```python
from build123d import *

# Parameters (mm, degrees)
BOSS_EXTRUDE1_DEPTH      = 4.7625
M4_CLEARANCE_HOLE1_D     = 4.5
M4_CLEARANCE_HOLE1_DEPTH = 50
M4_CLEARANCE_HOLE1_TIP   = 1.351936393


with BuildPart() as part:
    # Sketch1 → Boss-Extrude1 (new body)
    with BuildSketch(Plane(origin=(0, 0, 0), x_dir=(1, 0, 0), z_dir=(0, 1, 0))):
        with BuildLine():
            Line((-30, 60), (30, 60))
            ThreePointArc((30, 60), (51.213203436, 51.213203436), (60, 30))
            Line((60, 30), (60, -30))
            ThreePointArc((60, -30), (51.213203436, -51.213203436), (30, -60))
            Line((30, -60), (-30, -60))
            ThreePointArc((-30, -60), (-51.213203436, -51.213203436), (-60, -30))
            Line((-60, -30), (-60, 30))
            ThreePointArc((-60, 30), (-51.213203436, 51.213203436), (-30, 60))
        make_face()
    extrude(amount=BOSS_EXTRUDE1_DEPTH)

    # M4 Clearance Hole1
    with Locations(Plane(origin=(0, 4.7625, 0), x_dir=(1, 0, 0), z_dir=(0, 1, 0))):
        with Locations((0, 47.3)):
            Hole(M4_CLEARANCE_HOLE1_D / 2, depth=M4_CLEARANCE_HOLE1_DEPTH)
            with Locations((0, 0, -(M4_CLEARANCE_HOLE1_DEPTH + M4_CLEARANCE_HOLE1_TIP / 2))):  # 118° drill point
                Cone(0, M4_CLEARANCE_HOLE1_D / 2, M4_CLEARANCE_HOLE1_TIP, mode=Mode.SUBTRACT)


solid = part.part
```
Geometry: final body of the model. Coordinates: model frame, mm. Give positions to 0.01 mm unless a question says otherwise; leave off trailing zeros. Order: outer loops, then holes, each group sorted by start corner. A loop starts at its lowest first (then second) coordinate and runs counter-clockwise, first axis right, second up. Notation, with made-up numbers: M 8,-30.75 L 58,-30.75 A11 ccw 58,-9.75 Z; hole C -3,37.5 d1. An arc over 180 degrees is marked long. Answer as CSV lines item,"result". Start each with the question number.
1) Cut plane B-B (x = 0). Output: boundary loops of the cut face in (y, z).
2) Cut plane A-A (y = 3.5). Output: boundary loops of the cut face in (x, z), then the cut area to 3 significant figures.
3) First-contact query: P1, Ø1.5, axis at y = 2.5, z = 42.5, coming from the -X side. Flat tip, straight axial feed; report the tip coordinate or a pass-through.
4) Cut plane C-C (z = -47.3). Output: boundary loops of the cut face in (x, y), then the cut area to 3 significant figures.
5) Cut plane D-D (x = 47). Output: boundary loops of the cut face in (y, z).
6) Mould query, pull axis X, two halves, no side actions, for faces 1 (the cylindrical face through (51.445, 2.348, 50.979)), 2 (the cylindrical face through (-1.038, 2.348, -45.304)), 3 (the flat face through (0, 2, -60)). Classes: +X half, -X half, draft (parallel to the pull), parting line (faces both ways), or undercut.
7) Line query: line 1 (Z direction, x = 0, y = 2.9); line 2 (X direction, y = 2.9, z = -47.3); line 3 (Z direction, x = 1, y = 0.4). Output: solid intervals per line, ascending. Write a range as from..to.
Findings below:
1,outline,"M 0,-60 L 4.76,-60 L 4.76,-49.55 L 0,-49.55 Z; M 0,-45.05 L 4.76,-45.05 L 4.76,60 L 0,60 Z"
2,outline,"M -60,-30 A30 ccw -30,-60 L 30,-60 A30 ccw 60,-30 L 60,30 A30 ccw 30,60 L -30,60 A30 ccw -60,30 Z; hole C 0,-47.3 d4.5"
2,area,"13,600 mm²"
3,P1,"stops at x = -57.6"
4,outline,"M -54.51,0 L -2.25,0 L -2.25,4.76 L -54.51,4.76 Z; M 2.25,0 L 54.51,0 L 54.51,4.76 L 2.25,4.76 Z"
4,area,"498 mm²"
5,outline,"M 0,-54.72 L 4.76,-54.72 L 4.76,54.72 L 0,54.72 Z"
6,face 1,"+X half"
6,face 2,"undercut"
6,face 3,"draft"
7,line 1,"z = -60..-49.55, -45.05..60"
7,line 2,"x = -54.51..-2.25, 2.25..54.51"
7,line 3,"z = -60..-49.32, -45.28..60"
